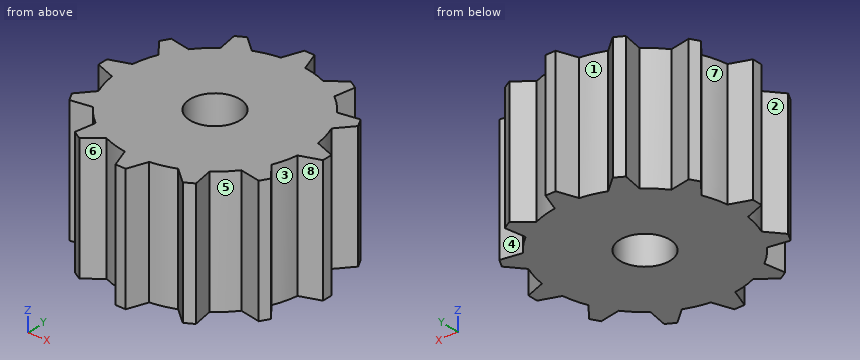
```python
from build123d import *

# Parameters (mm, degrees)
IZIM1_R                     = 7.5
Y_KSEKLIK_EKSTR_ZYON1_DEPTH = 5
Y_KSEKLIK_EKSTR_ZYON2_DEPTH = 5
IZIM3_R                     = 2
KES_EKSTR_ZYON1_DEPTH       = 11


with BuildPart() as part:
    # Çizim1 → Yükseklik-Ekstrüzyon1 (new body, symmetric)
    with BuildSketch(Plane.XY):
        Circle(IZIM1_R)
    extrude(amount=Y_KSEKLIK_EKSTR_ZYON1_DEPTH, both=True)

    # Çizim2 → Yükseklik-Ekstrüzyon2 (add, symmetric)
    with BuildSketch(Plane.XY):
        Polygon((-1.5, 6), (1.5, 6), (0.408089297, 9), (-0.408089297, 9), align=None)
        Polygon((4.146584302, 7.998273283), (1.700961894, 5.946152423), (4.299038106, 4.446152423), (4.853415698, 7.590183985), align=None)
        Polygon((7.590183985, 4.853415698), (4.446152423, 4.299038106), (5.946152423, 1.700961894), (7.998273283, 4.146584302), align=None)
        Polygon((9, 0.408089297), (6, 1.5), (6, -1.5), (9, -0.408089297), align=None)
        Polygon((7.998273283, -4.146584302), (5.946152423, -1.700961894), (4.446152423, -4.299038106), (7.590183985, -4.853415698), align=None)
        Polygon((4.853415698, -7.590183985), (4.299038106, -4.446152423), (1.700961894, -5.946152423), (4.146584302, -7.998273283), align=None)
        Polygon((0.408089297, -9), (1.5, -6), (-1.5, -6), (-0.408089297, -9), align=None)
        Polygon((-4.146584302, -7.998273283), (-1.700961894, -5.946152423), (-4.299038106, -4.446152423), (-4.853415698, -7.590183985), align=None)
        Polygon((-7.590183985, -4.853415698), (-4.446152423, -4.299038106), (-5.946152423, -1.700961894), (-7.998273283, -4.146584302), align=None)
        Polygon((-9, -0.408089297), (-6, -1.5), (-6, 1.5), (-9, 0.408089297), align=None)
        Polygon((-7.998273283, 4.146584302), (-5.946152423, 1.700961894), (-4.446152423, 4.299038106), (-7.590183985, 4.853415698), align=None)
        Polygon((-4.853415698, 7.590183985), (-4.299038106, 4.446152423), (-1.700961894, 5.946152423), (-4.146584302, 7.998273283), align=None)
    extrude(amount=Y_KSEKLIK_EKSTR_ZYON2_DEPTH, both=True)

    # Çizim3 → Kes-Ekstrüzyon1 (cut, through all)
    with BuildSketch(Plane.XY.offset(5)):
        Circle(IZIM3_R)
    extrude(amount=-KES_EKSTR_ZYON1_DEPTH, mode=Mode.SUBTRACT)


solid = part.part
```
Part model, mm, in its own coordinate system. Face numbers are marked on the shaded views. A direction names the side the tool comes from. Coordinates: 2 decimals unless noted, no trailing zeros. Order: outer loops, then holes, each group sorted by start corner. A loop starts at its lowest first (then second) coordinate and runs counter-clockwise, first axis right, second up. Notation, with made-up numbers: (40.5, 6.5) - (74.5, 6.5) arc R20 ccw to (74.5, 26.5) - close; hole circle Ø10 at (42.25, 22.5). An arc over 180 degrees is marked (long way). Return JSON: item names as keys, results as strings. Group by question number.
Item 1: Cut at C-C (y = 8.25). List the corners of the cut face in (x, z).
Item 2: Pin check, flat tips, straight feed: pin 1 (3 mm diameter, centred on x = 0, y = 0, fed in from +Z); pin 2 (6 mm diameter, centred on x = -2, z = -1.5, fed in from -Y); pin 3 (4 mm diameter, centred on x = -6, z = -0.5, fed in from -Y); pin 4 (6 mm diameter, centred on y = -4.5, z = -2, fed in from +X). Stop position of each tip, or through.
Item 3: Cut at A-A (y = 0). List the corners of the cut face in (x, z), plus the area to 3 significant figures.
Item 4: Which spindle directions (+Z, -Z, +X, -X, +Y, -Y) get a long thin tool onto all of the face, cutting with end or side? Do the marked faces 4, 5, 6, 7 and 8. Say none if no direction does.
Item 5: Drill centre lines: probe 1 along Y at (x, z) = (0, -1.5); probe 2 along X at (y, z) = (-7.5, -2.75); probe 3 along X at (y, z) = (2.75, 0.25). Where is each one in solid material? Low to high. Write a range as from..to.
Item 6: Pull direction X, two halves, no side cores. Call the marked faces 1, 2 and 3: pulls with the +X half, pulls with the -X half, needs draft (parallel to the pull), parting line crosses it, or undercut.
Check values:
{
 "1": {"outline": "(-0.68, -5) - (0.68, -5) - (0.68, 5) - (-0.68, 5) - close"},
 "2": {"pin 1": "passes through", "pin 2": "stops at y = -9", "pin 3": "stops at y = -8", "pin 4": "stops at x = 8"},
 "3": {"outline": "(-9, -5) - (-2, -5) - (-2, 5) - (-9, 5) - close; (2, -5) - (9, -5) - (9, 5) - (2, 5) - close", "area": "140 mm2"},
 "4": {"face 4": "+Z, -Z, +Y", "face 5": "+Z, -Z", "face 6": "+Z, -Z, -Y", "face 7": "+Z, -Z, -X", "face 8": "+Z, -Z, +X"},
 "5": {"probe 1": "y = -9..-2, 2..9", "probe 2": "x = -4.84..-3.55, -0.95..0.95, 3.55..4.84", "probe 3": "x = -6.98..6.98"},
 "6": {"face 1": "undercut", "face 2": "pulls with the -X half", "face 3": "pulls with the +X half"}
}
